The listing builds one solid part. Answer for the finished solid, in the listing's coordinates (mm). A direction names the side the tool comes from. Give positions to 0.01 mm unless a question says otherwise; leave off trailing zeros. Write each loop counter-clockwise with the first axis right and the second up, starting at its lowest first coordinate (ties: lowest second). Pieces come first, ordered by that corner, then holes. Notation, with made-up numbers: (4, -21) -> (17, -21) arc R36 ccw to (17, 17) -> close; hole circle Ø11 at (-15.75, 13.25). An arc over 180 degrees is marked (long way). Write each question's results on one line, items separated by ' | '. Start each with the question number.
from build123d import *

# Parameters (mm, degrees)
SKETCH_1_W      = 7.5
SKETCH_1_H      = 7
EXTRUDE_1_DEPTH = 2.5
SKETCH_2_R      = 2.25
EXTRUDE_2_DEPTH = 1.8
EXTRUDE_3_DEPTH = 0.5
SKETCH_4_W      = 1
SKETCH_4_H      = 2
EXTRUDE_4_DEPTH = 0.5
SKETCH_5_W      = 0.66
SKETCH_5_H      = 0.2
EXTRUDE_5_DEPTH = 3.6
SKETCH_6_W      = 0.5
SKETCH_6_H      = 0.5
EXTRUDE_6_DEPTH = 5.6


with BuildPart() as part:
    # 草图1 → 凸台-拉伸1 (new body)
    with BuildSketch(Plane.XY):
        Rectangle(SKETCH_1_W, SKETCH_1_H)
    extrude(amount=EXTRUDE_1_DEPTH)

    # 草图2 → 凸台-拉伸2 (add)
    with BuildSketch(Plane(origin=(0, 0, 0), x_dir=(-1, 0, 0), z_dir=(0, 0, -1))):
        Circle(SKETCH_2_R)
    extrude(amount=EXTRUDE_2_DEPTH)

    # 草图3 → 凸台-拉伸3 (add)
    with BuildSketch(Plane(origin=(3.75, 0, 0), x_dir=(0, 0, -1), z_dir=(1, 0, 0))):
        Polygon((0, 3.5), (0, -3.5), (-2.5, -3.5), (-6.35, -3.5), (-4.5, 3.5), align=None)
    extrude_3 = extrude(amount=-EXTRUDE_3_DEPTH)

    # 草图4 → 凸台-拉伸4 (add)
    with BuildSketch(Plane(origin=(3.75, 0, 0), x_dir=(0, 0, -1), z_dir=(1, 0, 0))):
        with Locations((-5.05, -4.5)):
            Rectangle(SKETCH_4_W, SKETCH_4_H)
    extrude_4 = extrude(amount=-EXTRUDE_4_DEPTH)

    # 镜向1: 凸台-拉伸3, 凸台-拉伸4 across plane
    add(extrude_3.mirror(Plane(origin=(0, 0, 0), x_dir=(0, 0, 1), z_dir=(1, 0, 0))))
    add(extrude_4.mirror(Plane(origin=(0, 0, 0), x_dir=(0, 0, 1), z_dir=(1, 0, 0))))

    # 草图5 → 凸台-拉伸5 (add)
    with BuildSketch(Plane.XZ.offset(3.5)):
        with Locations((-2.169711975, 2.55)):
            Rectangle(SKETCH_5_W, SKETCH_5_H)
        with Locations((2.169711975, 2.55)):
            Rectangle(SKETCH_5_W, SKETCH_5_H)
    extrude(amount=EXTRUDE_5_DEPTH)

    # 草图6 → 凸台-拉伸6 (add)
    with BuildSketch(Plane(origin=(0, 0, 0), x_dir=(-1, 0, 0), z_dir=(0, 0, -1))):
        with Locations((-3.5, -3.75)):
            Rectangle(SKETCH_6_W, SKETCH_6_H)
        with Locations((3.5, -3.75)):
            Rectangle(SKETCH_6_W, SKETCH_6_H)
    extrude(amount=-EXTRUDE_6_DEPTH)


solid = part.part
1. Section B-B (z = 3.25) is taken. Write down the section's boundary in (x, y).
2. Each of these flat-tipped pins is pushed along its axis until it touches: pin 1 Ø1.2 at (x, z) = (0.5, 1) entering from -Y; pin 2 Ø3 at (x, y) = (1, -1.5) entering from +Z. Where does it stop, or does it pass through?
3. Section D-D (x = 0) is taken. Write down the section's boundary in (y, z).
4. Consider probe 1 along X at (y, z) = (-2, 4.25); probe 2 along Y at (x, z) = (-3, 1.75); probe 3 along Z at (x, y) = (-2, 0.75). Determine where each line is inside the solid, lowest interval first. Write a range as [from, to].
5. A tool of negligible diameter and unlimited length cuts with its end or side. For faces 4 (the flat face through (0, 0, 2.5)), 5 (the flat face through (0.9, 2.3, 0)), 6 (the flat face through (-3.5, -0.05, 5.44)), from which of +Z, -Z, +X, -X, +Y, -Y can it reach the whole face along a straight path? Write none if from no direction.
6. Section A-A (y = -5) is taken. Write down the section's boundary in (x, z).
7. Section C-C (y = -6.5) is taken. Write down the section's boundary in (x, z).
8. The mould has two halves that part along X. Classify faces 1 (the flat face through (3.5, -0.05, 5.44)), 2 (the cylindrical face through (0.29, 2.23, -0.89)), 3 (the flat face through (0, -3.5, 1)): pulls with the +X half, pulls with the -X half, needs draft (parallel to the pull), parting line crosses it, or undercut.
Results:
1) outline: (-3.75, -4) -> (-3.25, -4) -> (-3.25, 3.5) -> (-3.75, 3.5) -> close; (3.25, -4) -> (3.75, -4) -> (3.75, 3.5) -> (3.25, 3.5) -> close
2) pin 1: stops at y = -3.5 | pin 2: stops at z = 2.5
3) outline: (-3.5, 0) -> (-2.25, 0) -> (-2.25, -1.8) -> (2.25, -1.8) -> (2.25, 0) -> (3.5, 0) -> (3.5, 2.5) -> (-3.5, 2.5) -> close
4) probe 1: x = [-3.75, -3.25], [3.25, 3.75] | probe 2: y = [-3.5, 3.5] | probe 3: z = [-1.8, 2.5]
5) face 4: +Z, +Y | face 5: -Z | face 6: +Z, +X, -X, +Y
6) outline: (-3.75, 4.55) -> (-3.25, 4.55) -> (-3.25, 5.55) -> (-3.75, 5.55) -> close; (-2.5, 2.45) -> (-1.84, 2.45) -> (-1.84, 2.65) -> (-2.5, 2.65) -> close; (1.84, 2.45) -> (2.5, 2.45) -> (2.5, 2.65) -> (1.84, 2.65) -> close; (3.25, 4.55) -> (3.75, 4.55) -> (3.75, 5.55) -> (3.25, 5.55) -> close
7) outline: (-2.5, 2.45) -> (-1.84, 2.45) -> (-1.84, 2.65) -> (-2.5, 2.65) -> close; (1.84, 2.45) -> (2.5, 2.45) -> (2.5, 2.65) -> (1.84, 2.65) -> close
8) face 1: needs draft | face 2: parting line crosses it | face 3: undercut
